The listing builds one solid part. Answer for the finished solid, in the listing's coordinates (mm). Face numbers are marked on the shaded views. Give positions to 0.01 mm unless a question says otherwise; leave off trailing zeros. Order: outer loops, then holes, each group sorted by start corner. A loop starts at its lowest first (then second) coordinate and runs counter-clockwise, first axis right, second up. Notation, with made-up numbers: (57.5, 42) - (84.5, 42) arc R20 ccw to (84.5, 63) - close; hole circle Ø2 at (-35, -40). An arc over 180 degrees is marked (long way). Answer in a Markdown table with one row per item.
from build123d import *

# Parameters (mm, degrees)
SKETCH1_W               = 34.5
SKETCH1_H               = 20
BOSS_EXTRUDE1_DEPTH     = 2
FILLET1_R               = 2
SKETCH2_W               = 16
SKETCH2_H               = 2.2
SKETCH2_W_2             = 2
SKETCH2_H_2             = 7.4
SKETCH2_H_3             = 26.2
SKETCH2_H_4             = 13.8
BOSS_EXTRUDE2_DEPTH     = 2
CUT_EXTRUDE1_DEPTH      = 1.9
CUT_EXTRUDE1_DEPTH_BACK = 1.9
SKETCH3_W               = 2.2
SKETCH3_H               = 2


with BuildPart() as part:
    # Sketch1 → Boss-Extrude1 (new body)
    with BuildSketch(Plane(origin=(0, 0, 0), x_dir=(0, 1, 0), z_dir=(0, 0, 1))):
        Rectangle(SKETCH1_W, SKETCH1_H)
    extrude(amount=BOSS_EXTRUDE1_DEPTH)

    # Fillet1
    fillet1_edges = [part.edges().sort_by_distance(p)[0] for p in [
        (-10, 0, 0),
        (10, 0, 0),
    ]]
    fillet(fillet1_edges, radius=FILLET1_R - 0.0001)  # a hair under: the kernel refuses the full size

    # Sketch2 → Boss-Extrude2 (add)
    with BuildSketch(Plane.XY.offset(2)):
        with Locations((0, 14.05)):
            Rectangle(SKETCH2_W, SKETCH2_H)
        with Locations((-7, -11.45)):
            Rectangle(SKETCH2_W_2, SKETCH2_H_2)
        with Locations((7, -2.05)):
            Rectangle(SKETCH2_W_2, SKETCH2_H_3)
        with Locations((-7, 4.15)):
            Rectangle(SKETCH2_W_2, SKETCH2_H_4)
    extrude(amount=BOSS_EXTRUDE2_DEPTH)

    # Sketch3 → Cut-Extrude1 (cut, two sides: drawn at the far end of the back side and taken through both)
    with BuildSketch(Plane.YZ.offset(-CUT_EXTRUDE1_DEPTH_BACK)):
        with Locations((14.05, 3)):
            Rectangle(SKETCH3_W, SKETCH3_H)
    extrude(amount=CUT_EXTRUDE1_DEPTH + CUT_EXTRUDE1_DEPTH_BACK, mode=Mode.SUBTRACT)


solid = part.part
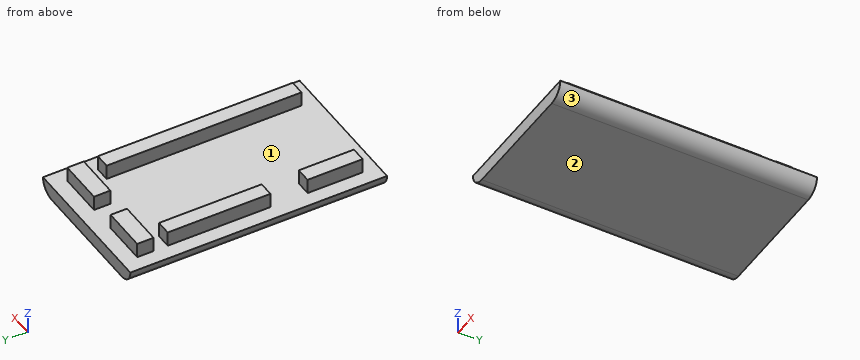
Item 1: Find section C-C on x = -7.5. Write down the section's boundary in (y, z).
Answer block:
| item | result |
|---|---|
| outline | (-17.25, 0) - (17.25, 0) - (17.25, 2) - (15.15, 2) - (15.15, 4) - (12.95, 4) - (12.95, 2) - (11.05, 2) - (11.05, 4) - (-2.75, 4) - (-2.75, 2) - (-7.75, 2) - (-7.75, 4) - (-15.15, 4) - (-15.15, 2) - (-17.25, 2) - close |
Item 2: Consider line 1 (Y direction, x = 7.75, z = 2.3); line 2 (X direction, y = 7.5, z = 2.15); line 3 (Z direction, x = -0.75, y = 12). Determine where each line is inside the solid, lowest interval first.
Answer block:
| item | result |
|---|---|
| line 1 | -15.15 to 11.05, 12.95 to 15.15 |
| line 2 | -8 to -6, 6 to 8 |
| line 3 | 0 to 2 |
Item 3: Find section D-D on x = 5.5. Write down the section's boundary in (y, z), then the cut area to 3 significant figures.
Answer block:
| item | result |
|---|---|
| outline | (-17.25, 0) - (17.25, 0) - (17.25, 2) - (15.15, 2) - (15.15, 4) - (12.95, 4) - (12.95, 2) - (-17.25, 2) - close |
| area | 73.4 mm² |
Item 4: Each of these flat-tipped pins is pushed along its axis until it touches: P1, Ø0.6, axis at x = -7, z = 3, coming from the +Y side; P2, Ø1.6, axis at x = -6, z = 3.5, coming from the -Y side; P3, Ø3, axis at x = 0, y = 9, coming from the +Z side. Where does it stop, or does it pass through?
Answer block:
| item | result |
|---|---|
| P1 | y = 15.15 |
| P2 | y = -15.15 |
| P3 | z = 2 |
Item 5: Determine the mould class of the marked faces 1, 2 and 3 for opening direction X: pulls with the +X half, pulls with the -X half, needs draft (parallel to the pull), parting line crosses it, or undercut.
Answer block:
| item | result |
|---|---|
| face 1 | undercut |
| face 2 | needs draft |
| face 3 | pulls with the +X half |
Item 6: Find section A-A on z = 2.9. Write down the section's boundary in (x, y).
Answer block:
| item | result |
|---|---|
| outline | (-8, -15.15) - (-6, -15.15) - (-6, -7.75) - (-8, -7.75) - close; (-8, -2.75) - (-6, -2.75) - (-6, 11.05) - (-8, 11.05) - close; (-8, 12.95) - (-1.9, 12.95) - (-1.9, 15.15) - (-8, 15.15) - close; (1.9, 12.95) - (8, 12.95) - (8, 15.15) - (1.9, 15.15) - close; (6, -15.15) - (8, -15.15) - (8, 11.05) - (6, 11.05) - close |
